Answer from the drawing. Dimensions are ordinates in mm from the lowest x, y and z of the part. Round coordinates to 2 decimals unless told otherwise and drop trailing zeros. Write each loop counter-clockwise with the first axis right and the second up, starting at its lowest first coordinate (ties: lowest second). Pieces come first, ordered by that corner, then holes. Notation, with made-up numbers: (-20.5, -33.75) - (4.5, -33.75) arc R5 ccw to (4.5, -24.75) - close; hole circle Ø5 at (78.25, -39.5). An arc over 180 degrees is marked (long way). Use a Markdown table: item, result. Add a question column.
1) Each of these flat-tipped pins is pushed along its axis until it touches: P1, Ø2, axis at y = 46.5, z = 2, coming from the +X side; P2, Ø1.2, axis at x = 67, z = 2, coming from the +Y side; P3, Ø1.1, axis at y = 42.5, z = 0.5, coming from the -X side; P4, Ø2, axis at x = 17.5, y = 7.5, coming from the -Z side. Where does it stop, or does it pass through?
2) Determine the mould class of the marked faces 1 and 2 for opening direction Y: +Y half, -Y half, draft (parallel to the pull), parting line (faces both ways), or undercut.
3) A cutting plane is placed at A-A (y = 29). Give the vertices of the cut face in (x, z), then the cut area to 4 significant figures.
4) A cutting plane is placed at C-C (z = 2.6). Give the vertices of the cut face in (x, y).
5) A cutting plane is placed at B-B (y = 53.5). Give the vertices of the cut face in (x, z).
6) Find the intervals of material crossed by probe 1 along X at (y, z) = (29, 1.15); probe 2 along X at (y, z) = (50.5, 3.5); probe 3 along Y at (x, z) = (38, 0.75), in increasing order. Write a range as from..to.
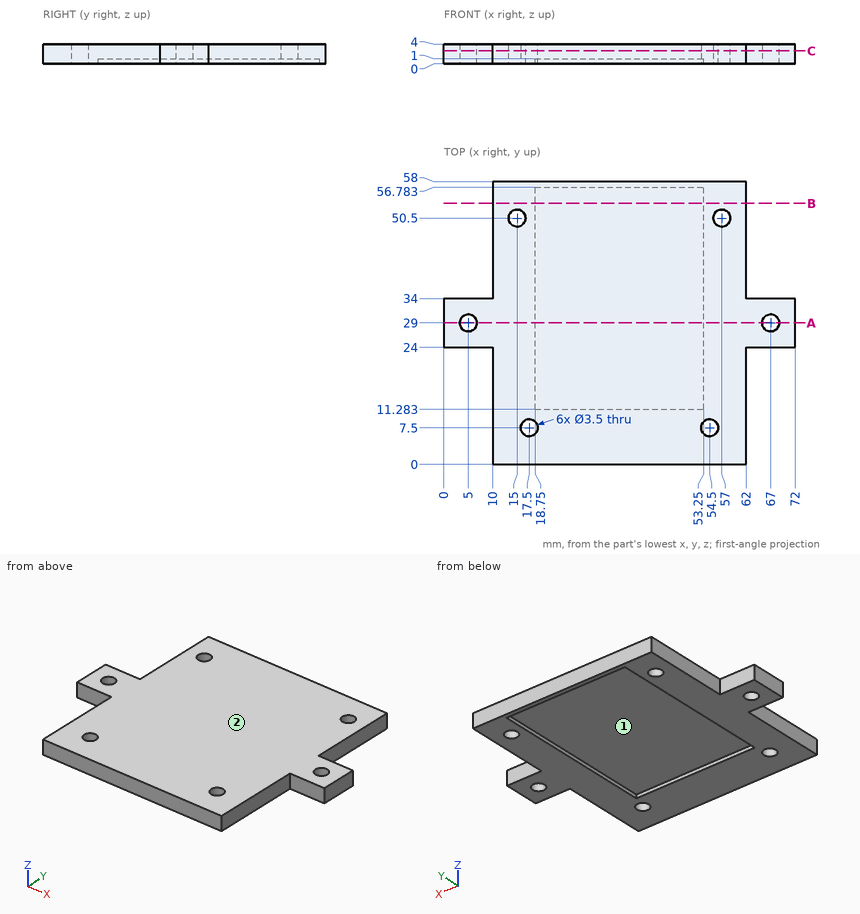
Entries:
| question | item | result |
|---|---|---|
| 1 | P1 | stops at x = 62 |
| 1 | P2 | stops at y = 34 |
| 1 | P3 | stops at x = 10 |
| 1 | P4 | passes through |
| 2 | face 1 | undercut |
| 2 | face 2 | draft |
| 3 | outline | (0, 0) - (3.25, 0) - (3.25, 4) - (0, 4) - close; (6.75, 0) - (18.75, 0) - (18.75, 1) - (53.25, 1) - (53.25, 0) - (65.25, 0) - (65.25, 4) - (6.75, 4) - close; (68.75, 0) - (72, 0) - (72, 4) - (68.75, 4) - close |
| 3 | area | 225.5 mm² |
| 4 | outline | (0, 24) - (10, 24) - (10, 0) - (62, 0) - (62, 24) - (72, 24) - (72, 34) - (62, 34) - (62, 58) - (10, 58) - (10, 34) - (0, 34) - close; hole circle Ø3.5 at (5, 29); hole circle Ø3.5 at (15, 50.5); hole circle Ø3.5 at (17.5, 7.5); hole circle Ø3.5 at (54.5, 7.5); hole circle Ø3.5 at (57, 50.5); hole circle Ø3.5 at (67, 29) |
| 5 | outline | (10, 0) - (18.75, 0) - (18.75, 1) - (53.25, 1) - (53.25, 0) - (62, 0) - (62, 4) - (10, 4) - close |
| 6 | probe 1 | x = 0..3.25, 6.75..65.25, 68.75..72 |
| 6 | probe 2 | x = 10..13.25, 16.75..55.25, 58.75..62 |
| 6 | probe 3 | y = 0..11.28, 56.78..58 |
